Input: part model. Units: mm. Frame: model coordinates. Face numbers are marked on the shaded views. Round coordinates to 2 decimals unless told otherwise and drop trailing zeros. Loops run counter-clockwise (first coordinate to the right, second up) from the corner with the lowest first, then second, coordinate; pieces in that order, holes last. Notation, with made-up numbers: M 74,75.5 L 106,75.5 A13 ccw 106,98.5 Z; hole C 76.25,3.5 d9. An arc over 180 degrees is marked long. Return JSON: item names as keys, results as strings. Group by question number.
1) Contact query for flat-ended pins moving along their axis: P1, Ø5, axis at x = 2, y = 15.5, coming from the +Z side; P2, Ø24.5, axis at y = 9.5, z = -6.5, coming from the -X side; P3, Ø8, axis at y = 17, z = -22, coming from the +X side. Output: stop coordinate, or through.
2) Mould query, pull axis Z, two halves, no side actions, for the marked faces 1, 2 and 3. Classes: +Z half, -Z half, draft (parallel to the pull), parting line (faces both ways), or undercut.
3) Section A-A (x = 4). Output: boundary loops of the cut face in (y, z).
4) Material intervals for line 1 (Z direction, x = 3.1, y = 0); line 2 (X direction, y = -29, z = -24); line 3 (X direction, y = -32, z = -11), sorted ascending. Write a range as from..to.
5) Section C-C (y = -35). Output: boundary loops of the cut face in (x, z), plus the area to 3 significant figures.
6) Section B-B (z = 32.5). Output: boundary loops of the cut face in (x, y), plus the area to 3 significant figures.
Autodesk Inventor part; units mm, degrees
ref_plane "YZ Plane" through (0, 0, 0) normal (1, 0, 0) x (0, 1, 0)
ref_plane "XZ Plane" through (0, 0, 0) normal (0, 1, 0) x (-1, 0, 0)
ref_plane "XY Plane" through (0, 0, 0) normal (0, 0, 1) x (1, 0, 0)
sketch "Sketch1" plane through (0, 0, 0) normal (0, 0, 1) x (1, 0, 0)
  line L0 (0, 0) -> (0, 37.5)
  line L1 (0, 37.5) -> (7.5, 37.5)
  line L2 (7.5, 37.5) -> (7.5, 40.5)
  line L3 (7.5, 40.5) -> (9.5, 40.5)
  line L4 (9.5, 40.5) -> (9.5, 31)
  line L5 (151.3726, 0) -> (0, 0)
  line L6 (9.5, 31) -> (11, 31)
  arc A0 (16, 0) -> (11, 31) centre (-75.9938, 1.0655) ccw
  line L7 (0, 34) -> (9.5, 34) construction
  dimension "d1" = 2
  dimension "d2" = 7.5
  dimension "d4" = 75
  dimension "d5" = 81
  dimension "d6" = 1.5
  dimension "d7" = 92
  dimension "d8" = 68
  dimension "d9" = 16
  dimension "d10" = 62
revolve "Revolution1" add sketch "Sketch1" angle 360 about axis through (151.3726, 0, 0) along (-1, 0, 0)
sketch "Sketch2" plane through (0, 0, 0) normal (-1, 0, 0) x (0, 0, 1)
  circle A0 centre (0, 0) radius 37.5
hole "Hole1" at (0, 0, 0) direction (1, 0, 0) diameter 68 depth 5.5
sketch "Sketch3" plane through (5.5, 0, 0) normal (-1, 0, 0) x (0, 0, 1)
  circle A0 centre (0, 0) radius 31
hole "Hole2" at (5.5, 0, 0) direction (1, 0, 0) diameter 3.242 end through all
properties part number "130 part 2" material "Aluminum 6061-AHC"
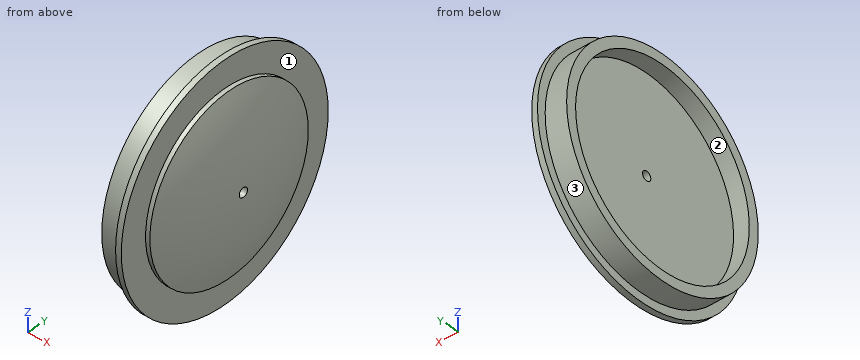
Returned:
{
 "1": {"P1": "stops at z = 35.17", "P2": "stops at x = 5.5", "P3": "stops at x = 13.15"},
 "2": {"face 1": "draft", "face 2": "undercut", "face 3": "parting line"},
 "3": {"outline": "C 0,0 d75; hole C 0,0 d68"},
 "4": {"line 1": "z = -37.5..-34, 34..37.5", "line 2": "x = 7.5..9.5", "line 3": "x = 5.5..9.5"},
 "5": {"outline": "M 0,-13.46 L 7.5,-13.46 L 7.5,-20.38 L 9.5,-20.38 L 9.5,20.38 L 7.5,20.38 L 7.5,13.46 L 0,13.46 Z", "area": "283 mm^2"},
 "6": {"outline": "M 0,-18.71 L 7.5,-18.71 L 7.5,-24.17 L 9.5,-24.17 L 9.5,24.17 L 7.5,24.17 L 7.5,18.71 L 0,18.71 L 0,9.99 L 5.5,9.99 L 5.5,-9.99 L 0,-9.99 Z", "area": "267 mm^2"}
}
